Could you check a few things on this model? Use its own coordinates, in mm. A direction names the side the tool comes from. Coordinates: 2 decimals unless noted, no trailing zeros. Order: outer loops, then holes, each group sorted by start corner. A loop starts at its lowest first (then second) coordinate and runs counter-clockwise, first axis right, second up. Notation, with made-up numbers: (80, 44) - (93, 44) arc R15 ccw to (93, 53) - close; hole circle Ø1 at (66.25, 69). An arc over 180 degrees is marked (long way). One line per item, written item: value. Start each with the question number.
from build123d import *

# Parameters (mm, degrees)
SKETCH1_R           = 95
BOSS_EXTRUDE1_DEPTH = 6.7
SKETCH2_W           = 6.7
SKETCH2_H           = 20
CUT_EXTRUDE3_DEPTH  = 6.7
SKETCH3_R           = 8
CUT_EXTRUDE4_DEPTH  = 3.35


with BuildPart() as part:
    # Sketch1 → Boss-Extrude1 (new body)
    with BuildSketch(Plane(origin=(0, 0, 0), x_dir=(1, 0, 0), z_dir=(0, 1, 0))):
        with Locations(Location((0, 0, 0), (0, 0, 270))):
            Circle(SKETCH1_R)
    extrude(amount=BOSS_EXTRUDE1_DEPTH)

    # Sketch2 → Cut-Extrude3 (cut)
    with BuildSketch(Plane(origin=(0, 6.7, 0), x_dir=(1, 0, 0), z_dir=(0, 1, 0))):
        with BuildLine():
            Line((5, -8), (-5, -8))
            Line((-5, -8), (-4, -20))
            ThreePointArc((-4, -20), (0, -24), (4, -20))
            Line((4, -20), (5, -8))
        make_face()
        Polygon((87.936978657, 54.638685103), (70.616470581, 44.638685103), (73.966470581, 38.836314897), (91.286978657, 48.836314897), align=None)
        Polygon((69.078696797, -77.113110259), (56.222944603, -61.792221397), (51.090446834, -66.098898382), (63.946199028, -81.419787244), align=None)
        Polygon((102.484703638, -14.669139211), (82.788548578, -11.196175658), (81.625105788, -17.794387603), (101.321260848, -21.267351157), align=None)
        with Locations((0, -93.475)):
            Rectangle(SKETCH2_W, SKETCH2_H)
        Polygon((-63.946199028, -81.419787244), (-51.090446834, -66.098898382), (-56.222944603, -61.792221397), (-69.078696797, -77.113110259), align=None)
        Polygon((-101.321260848, -21.267351157), (-81.625105788, -17.794387603), (-82.788548578, -11.196175658), (-102.484703638, -14.669139211), align=None)
        Polygon((-91.286978657, 48.836314897), (-73.966470581, 38.836314897), (-70.616470581, 44.638685103), (-87.936978657, 54.638685103), align=None)
    extrude(amount=-CUT_EXTRUDE3_DEPTH, mode=Mode.SUBTRACT)

    # Sketch3 → Cut-Extrude4 (cut)
    with BuildSketch(Plane(origin=(0, 6.7, 0), x_dir=(1, 0, 0), z_dir=(0, 1, 0))):
        with Locations((0, -20)):
            Circle(SKETCH3_R)
    extrude(amount=-CUT_EXTRUDE4_DEPTH, mode=Mode.SUBTRACT)


solid = part.part
Q1. I want a section at C-C on z = 47. Please give me the cut outline in (x, y).
Q2. I want a section at D-D on x = -20.5. Please give me the cut outline in (y, z).
Q3. We'd pull the mould along X, two halves only. Please class faces 1 (the flat face through (87.192, 3.397, 18.776)), 2 (the flat face through (54.7, 3.4, 70.4)), 3 (the cylindrical face through (-82.5, 3.3, 47.1)): +X half, -X half, draft (parallel to the pull), parting line (faces both ways), or undercut.
Q4. Which directions (+Z, -Z, +X, -X, +Y, -Y) give clear straight access to the entire face, cutting with the end or side of a thin tool? Please do faces 4 (the flat face through (-82.2, 3.4, 14.54)), 5 (the cylindrical face through (1.35, 3.3, -94.99)), 6 (the flat face through (-3.35, 3, 89)).
Q5. If I drill on L1, parallel to X at y = 5.5, z = 20; L2, parallel to X at y = 4.25, z = 82; L3, parallel to Z at x = -40, y = 3.5, over which ranges is the centre line in solid material (lowest first)?
Q6. I want a section at B-B on x = 0. Please give me the cut outline in (y, z) (3 decimals), then the cut area to 3 significant figures.
Q7. I'm going to push flat-ended pins straight in: pin 1 (3 mm diameter, centred on y = 6, z = -52, fed in from +X); pin 2 (3 mm diameter, centred on x = -37.5, y = 4, fed in from +Z); pin 3 (2 mm diameter, centred on x = 1, y = 5, fed in from +Z) (3 decimals). Where does each tip first touch, or does it pass through?
Values follow:
1. outline: (-82.56, 0) - (82.56, 0) - (82.56, 6.7) - (-82.56, 6.7) - close
2. outline: (0, -92.76) - (6.7, -92.76) - (6.7, 92.76) - (0, 92.76) - close
3. face 1: +X half
3. face 2: undercut
3. face 3: -X half
4. face 4: +Y, -Y
4. face 5: -Z, +Y, -Y
4. face 6: +Z, +Y, -Y
5. L1: x = -92.87 to -8, 8 to 92.87
5. L2: x = -47.97 to 47.97
5. L3: z = -86.17 to 86.17
6. outline: (0, -95) - (6.7, -95) - (6.7, 8) - (0, 8) - close; (0, 24) - (3.35, 24) - (3.35, 28) - (6.7, 28) - (6.7, 83.475) - (0, 83.475) - close
6. area: 1,080 mm^2
7. pin 1: stops at x = 80.47
7. pin 2: stops at z = 87.91
7. pin 3: stops at z = 83.475
